```python
from build123d import *

# Parameters (mm, degrees)
SKETCH1_R           = 41
BOSS_EXTRUDE1_DEPTH = 3.5
SKETCH2_R           = 37.5
BOSS_EXTRUDE2_DEPTH = 3
SKETCH4_R           = 31.5
CUT_EXTRUDE3_DEPTH  = 3
CUT_EXTRUDE4_DEPTH  = 21
FILLET1_R           = 1.5


with BuildPart() as part:
    # Sketch1 → Boss-Extrude1 (new body)
    with BuildSketch(Plane.XY):
        Circle(SKETCH1_R)
    extrude(amount=BOSS_EXTRUDE1_DEPTH)

    # Sketch2 → Boss-Extrude2 (add)
    with BuildSketch(Plane.XY):
        Circle(SKETCH2_R)
    extrude(amount=-BOSS_EXTRUDE2_DEPTH)

    # Sketch4 → Cut-Extrude3 (cut)
    with BuildSketch(Plane.XY.offset(3.5)):
        Circle(SKETCH4_R)
    extrude(amount=-CUT_EXTRUDE3_DEPTH, mode=Mode.SUBTRACT)

    # Sketch5 → Cut-Extrude4 (cut)
    with BuildSketch(Plane.XY.offset(3.5)):
        with BuildLine():
            Line((-16, 22), (-16, 6))
            ThreePointArc((-16, 6), (-12, 2), (-8, 6))
            Line((-8, 6), (-8, 22))
            ThreePointArc((-8, 22), (-12, 26), (-16, 22))
        make_face()
        with BuildLine():
            Line((-8, -22), (-8, -6))
            ThreePointArc((-8, -6), (-12, -2), (-16, -6))
            Line((-16, -6), (-16, -22))
            ThreePointArc((-16, -22), (-12, -26), (-8, -22))
        make_face()
        with BuildLine():
            Line((16, -22), (16, -6))
            ThreePointArc((16, -6), (12, -2), (8, -6))
            Line((8, -6), (8, -22))
            ThreePointArc((8, -22), (12, -26), (16, -22))
        make_face()
        with BuildLine():
            Line((16, 22), (16, 6))
            ThreePointArc((16, 6), (12, 2), (8, 6))
            Line((8, 6), (8, 22))
            ThreePointArc((8, 22), (12, 26), (16, 22))
        make_face()
    extrude(amount=-CUT_EXTRUDE4_DEPTH, mode=Mode.SUBTRACT)

    # Fillet1
    fillet1_edges = [part.edges().sort_by_distance(p)[0] for p in [
        (-31.5, 0, 0.5),
        (-31.5, 0, 3.5),
        (-41, 0, 3.5),
    ]]
    fillet(fillet1_edges, radius=FILLET1_R - 0.0001)  # a hair under: the kernel refuses the full size


solid = part.part
```
Could you check a few things on this model? Use its own coordinates, in mm. A direction names the side the tool comes from. Round coordinates to 2 decimals unless told otherwise and drop trailing zeros. Loops run counter-clockwise (first coordinate to the right, second up) from the corner with the lowest first, then second, coordinate; pieces in that order, holes last.
Q1. On a 3-axis mill with a long thin cutter (end or side, diameter ignored), from which of +Z, -Z, +X, -X, +Y, -Y can I reach the whole of each face in a straight line? I mean faces 1 (the flat face through (0, 0, 0.5)), 2 (the flat face through (16, 14, -1)). Say none if no direction works.
Q2. I want a section at B-B (y = -9.5). Give the number of separate pieces and of enclosed holes in the cut face, and give its area (3 significant figures).
Q3. Please list where these lines run through material, in increasing order: L1, parallel to Y at x = 0, z = 2; L2, parallel to X at y = -18, z = -1.75; L3, parallel to X at y = -13, z = -2.25.
Q4. I want a section at A-A (z = -1.25). Write out the boundary of the cut face in (x, y).
Q5. For P1, Ø1, axis at x = 2.5, y = -9, coming from the +Z side; P2, Ø3, axis at y = -11.5, z = -2, coming from the +X side; P3, Ø1.8, axis at y = -17, z = -0.5, coming from the -X side, each with a flat end and sliding along its axis, tell me the tip position at first contact or that it passes through.
Q6. Thinking about a two-plate mould opening in X: for faces 3 (the cylindrical face through (-4.88, 37.18, -1.48)), 4 (the cylindrical face through (12, -2, -1)), which applies, pulls with the +X half, pulls with the -X half, needs draft (parallel to the pull), parting line crosses it, or undercut?
Answer below:
1. face 1: +Z
1. face 2: +Z, -Z
2. separate pieces: 3
2. enclosed holes: 0
2. area: 260 mm2
3. L1: y = -41 to -31.5, 31.5 to 41
3. L2: x = -32.9 to -16, -8 to 8, 16 to 32.9
3. L3: x = -35.17 to -16, -8 to 8, 16 to 35.17
4. outline: circle Ø75 at (0, 0); hole (-16, -22) arc R4 ccw to (-8, -22) - (-8, -6) arc R4 ccw to (-16, -6) - close; hole (-16, 6) arc R4 ccw to (-8, 6) - (-8, 22) arc R4 ccw to (-16, 22) - close; hole (8, -22) arc R4 ccw to (16, -22) - (16, -6) arc R4 ccw to (8, -6) - close; hole (8, 6) arc R4 ccw to (16, 6) - (16, 22) arc R4 ccw to (8, 22) - close
5. P1: stops at z = 0.5
5. P2: stops at x = 36.14
5. P3: stops at x = -37.64
6. face 3: parting line crosses it
6. face 4: undercut
